Build history of the part. All positions in model axes, mm. A direction names the side the tool comes from. Round coordinates to 2 decimals unless told otherwise and drop trailing zeros. Write each loop counter-clockwise with the first axis right and the second up, starting at its lowest first coordinate (ties: lowest second). Pieces come first, ordered by that corner, then holes.
from build123d import *

# Parameters (mm, degrees)
SKETCH1_R                = 38.1
CENTERHUB_DEPTH          = 20.6375
RIB_DEPTH                = 3.175
LIGHTENING_HOLE_DEPTH    = 21.6375
FILLET1_R                = 6.35
CIRPATTERN1_COUNT        = 2
FILLET1_OF_CIRPATTERN1_R = 6.35
SKETCH5_R                = 19.05
THRU_HOLE_DEPTH          = 21.6375
THRU_HOLE_DEPTH_BACK     = 21.6375


with BuildPart() as part:
    # Sketch1 → CenterHub (new body, symmetric)
    with BuildSketch(Plane.XY):
        Circle(SKETCH1_R)
    extrude(amount=CENTERHUB_DEPTH, both=True)

    # Sketch2 → Rim and Web (revolve)
    with BuildSketch(Plane(origin=(0, 0, 0), x_dir=(0, 0, -1), z_dir=(1, 0, 0))):
        Polygon((-6.35, 0), (6.35, 0), (6.35, 165.1), (19.05, 165.1), (19.05, 177.8), (-19.05, 177.8), (-19.05, 165.1), (-6.35, 165.1), align=None)
    revolve(axis=Axis((0, 0, 0), (0, 0, -1)))

    # Sketch3 → Rib (add, symmetric)
    with BuildSketch(Plane(origin=(0, 0, 0), x_dir=(1, 0, 0), z_dir=(0, 1, 0))):
        Polygon((0, -19.05), (132.747036773, -19.05), (167.64, -6.35), (167.64, 6.35), (132.747036773, 19.05), (0, 19.05), align=None)
    rib = extrude(amount=RIB_DEPTH, both=True)

    # Sketch4 → Lightening hole (cut, symmetric)
    with BuildSketch(Plane.XY):
        with BuildLine():
            Line((-151.204687427, -19.05), (-53.881536726, -19.05))
            ThreePointArc((-53.881536726, -19.05), (0, -57.15), (53.881536726, -19.05))
            Line((53.881536726, -19.05), (151.204687427, -19.05))
            ThreePointArc((151.204687427, -19.05), (0, -152.4), (-151.204687427, -19.05))
        make_face()
    lightening_hole = extrude(amount=LIGHTENING_HOLE_DEPTH, both=True, mode=Mode.SUBTRACT)

    # Fillet1
    fillet1_edges = [part.edges().sort_by_distance(p)[0] for p in [
        (151.204687427, -19.05, 0),
        (-151.204687427, -19.05, 0),
        (-53.881536726, -19.05, 0),
        (53.881536726, -19.05, 0),
    ]]
    fillet(fillet1_edges, radius=FILLET1_R)

    # CirPattern1: Rib, Lightening hole ×2 about axis
    cirpattern1_axis = Axis((0, 0, 0), (0, 0, 1))
    for i in range(1, CIRPATTERN1_COUNT):
        add(rib.rotate(cirpattern1_axis, i * 360 / CIRPATTERN1_COUNT))
        add(lightening_hole.rotate(cirpattern1_axis, i * 360 / CIRPATTERN1_COUNT), mode=Mode.SUBTRACT)

    # Fillet1 of CirPattern1
    fillet1_of_cirpattern1_edges = [part.edges().sort_by_distance(p)[0] for p in [
        (-151.204687427, 19.05, 0),
        (151.204687427, 19.05, 0),
        (53.881536726, 19.05, 0),
        (-53.881536726, 19.05, 0),
    ]]
    fillet(fillet1_of_cirpattern1_edges, radius=FILLET1_OF_CIRPATTERN1_R)

    # Sketch5 → Thru hole (cut, two sides)
    with BuildSketch(Plane.XY) as thru_hole_sk:
        Circle(SKETCH5_R)
    extrude(amount=THRU_HOLE_DEPTH, mode=Mode.SUBTRACT)
    extrude(thru_hole_sk.sketch, amount=-THRU_HOLE_DEPTH_BACK, mode=Mode.SUBTRACT)


solid = part.part
1) Pin check, flat tips, straight feed: pin 1 Ø14 at (x, z) = (-103.5, 13.5) entering from -Y; pin 2 Ø10 at (x, z) = (97.5, -10) entering from -Y; pin 3 Ø14 at (x, z) = (96, -3) entering from +Y; pin 4 Ø3 at (x, y) = (-126.5, 128.5) entering from -Z. Stop position of each tip, or through.
Results:
pin 1: stops at y = -149.33
pin 2: stops at y = -151.84
pin 3: stops at y = 153.92
pin 4: passes through
2) Wall check: L1, parallel to X at y = -52.5, z = 3; L2, parallel to Y at x = 35, z = -8; L3, parallel to X at y = -45.5, z = 0. Give the ranges that are in metal, low to high.
Results:
L1: x = -169.87 to -143.07, -22.58 to 22.58, 143.07 to 169.87
L2: y = -174.32 to -161.35, -15.05 to 15.05, 161.35 to 174.32
L3: x = -171.88 to -145.45, -34.58 to 34.58, 145.45 to 171.88
3) Which spindle directions (+Z, -Z, +X, -X, +Y, -Y) get a long thin tool onto all of the face, cutting with end or side? Do faces 1 (the flat face through (-102, -19.05, 0)), 2 (the flat face through (101, 3.175, -13)), 3 (the flat face through (1, 54, 6.35)). Say none if no direction does.
Results:
face 1: +Z, -Z
face 2: -Z
face 3: +Z
4) Slice it at D-D (y = -134). Write the cut outline in (x, z).
Results:
outline: (-116.86, -19.05) - (-96.45, -19.05) - (-96.45, -6.35) - (-72.59, -6.35) - (-72.59, 6.35) - (-96.45, 6.35) - (-96.45, 19.05) - (-116.86, 19.05) - close; (72.59, -6.35) - (96.45, -6.35) - (96.45, -19.05) - (116.86, -19.05) - (116.86, 19.05) - (96.45, 19.05) - (96.45, 6.35) - (72.59, 6.35) - close
5) Slice it at C-C (x = -111). Write the cut outline in (y, z) (3 decimals).
Results:
outline: (-138.895, -19.05) - (-122.217, -19.05) - (-122.217, -6.35) - (-104.426, -6.35) - (-104.426, 6.35) - (-122.217, 6.35) - (-122.217, 19.05) - (-138.895, 19.05) - close; (-19.05, -6.35) - (-3.175, -6.35) - (-3.175, -19.05) - (3.175, -19.05) - (3.175, -6.35) - (19.05, -6.35) - (19.05, 6.35) - (3.175, 6.35) - (3.175, 19.05) - (-3.175, 19.05) - (-3.175, 6.35) - (-19.05, 6.35) - close; (104.426, -6.35) - (122.217, -6.35) - (122.217, -19.05) - (138.895, -19.05) - (138.895, 19.05) - (122.217, 19.05) - (122.217, 6.35) - (104.426, 6.35) - close
6) Slice it at B-B (y = 52.5). Write the cut outline in (x, z), plus the area to 3 significant figures.
Results:
outline: (-169.87, -19.05) - (-156.53, -19.05) - (-156.53, -6.35) - (-143.07, -6.35) - (-143.07, 6.35) - (-156.53, 6.35) - (-156.53, 19.05) - (-169.87, 19.05) - close; (-22.58, -6.35) - (22.58, -6.35) - (22.58, 6.35) - (-22.58, 6.35) - close; (143.07, -6.35) - (156.53, -6.35) - (156.53, -19.05) - (169.87, -19.05) - (169.87, 19.05) - (156.53, 19.05) - (156.53, 6.35) - (143.07, 6.35) - close
area: 1,930 mm2
7) Slice it at A-A (x = 0). Count the separate pieces of the cut face and the enclosed holes in it, plus the area to 3 significant figures.
Results:
separate pieces: 4
enclosed holes: 0
area: 3,350 mm2
8) Mould opens along X. For faces 4 (the cylindrical face through (53.41, 169.59, 0.27)), 5 (the flat face through (-101, 3.175, -13)) say: released by +X, released by -X, zero draft, split by the parting line, or undercut.
Results:
face 4: split by the parting line
face 5: undercut
